Here's how the part is built. I have some questions about the finished solid (model axes, mm). Face numbers are marked on the shaded views. A direction names the side the tool comes from. Give positions to 0.01 mm unless a question says otherwise; leave off trailing zeros. Write each loop counter-clockwise with the first axis right and the second up, starting at its lowest first coordinate (ties: lowest second). Pieces come first, ordered by that corner, then holes. Notation, with made-up numbers: (62, -37.5) - (98, -37.5) arc R6 cw to (98, -32.5) - close; hole circle Ø9 at (33.25, 88.5). An arc over 180 degrees is marked (long way). Write each question's results on one line, items separated by ' | '. Start each with the question number.
Item 1: Which directions (+Z, -Z, +X, -X, +Y, -Y) give clear straight access to the entire face, cutting with the end or side of a thin tool? Please do the marked faces 1 and 2.
Item 2: We'd pull the mould along X, two halves only. Please class the marked faces 3, 4 and 5: +X half, -X half, draft (parallel to the pull), parting line (faces both ways), or undercut.
Item 3: Suppose I cut it at A-A on x = 0. List the corners of the cut face in (y, z) for me.
Item 4: Suppose I cut it at C-C on y = 13.5. List the corners of the cut face in (x, z) for me, then the cut area to 3 significant figures.
Item 5: Suppose I cut it at B-B on z = 0. List the corners of the cut face in (x, y) for me.
Item 6: Will these pins go through, and if not, where does the flat tip stop? P1, Ø4, axis at y = 7.5, z = -1.5, coming from the +X side; P2, Ø8, axis at x = -4, y = 35, coming from the +Z side; P3, Ø6, axis at x = 6.5, z = 5.5, coming from the -Y side; P4, Ø2.5, axis at x = 7, z = 0, coming from the -Y side.
Item 7: Suppose I cut it at D-D on x = 7.5. List the corners of the cut face in (y, z) for me, then the cut area to 3 significant figures.
Item 8: Please list where these lines run through material, in increasing order: line 1 along X through (y, z) = (42.1, 0); line 2 along X through (y, z) = (12, 0); line 3 along Y through (x, z) = (5.75, -8).
```python
from build123d import *

# Parameters (mm, degrees)
SKETCH1_R           = 1.5
BOSS_EXTRUDE1_DEPTH = 40
SKETCH2_R           = 10
SKETCH2_R_2         = 1.6
SKETCH2_R_3         = 1.5
BOSS_EXTRUDE2_DEPTH = 3


with BuildPart() as part:
    # Sketch1 → Boss-Extrude1 (new body)
    with BuildSketch(Plane(origin=(0, 0, 0), x_dir=(1, 0, 0), z_dir=(0, 1, 0))):
        with BuildLine():
            Line((2, 2.236067977), (2, -2.236067977))
            ThreePointArc((2, -2.236067977), (-3, 0), (2, 2.236067977))
        make_face()
        with Locations(Location((0, 0, 0), (0, 0, 270))):
            Circle(SKETCH1_R, mode=Mode.SUBTRACT)
    extrude(amount=BOSS_EXTRUDE1_DEPTH)

    # Sketch2 → Boss-Extrude2 (add)
    with BuildSketch(Plane(origin=(0, 40, 0), x_dir=(1, 0, 0), z_dir=(0, 1, 0))):
        with Locations(Location((0, 0, 0), (0, 0, 270))):
            Circle(SKETCH2_R)
        with Locations(Location((-7, 0, 0), (0, 0, 270))):
            Circle(SKETCH2_R_2, mode=Mode.SUBTRACT)
        with Locations(Location((7, 0, 0), (0, 0, 270))):
            Circle(SKETCH2_R_2, mode=Mode.SUBTRACT)
        with Locations(Location((0, 0, 0), (0, 0, 270))):
            Circle(SKETCH2_R_3, mode=Mode.SUBTRACT)
    extrude(amount=BOSS_EXTRUDE2_DEPTH)


solid = part.part
```
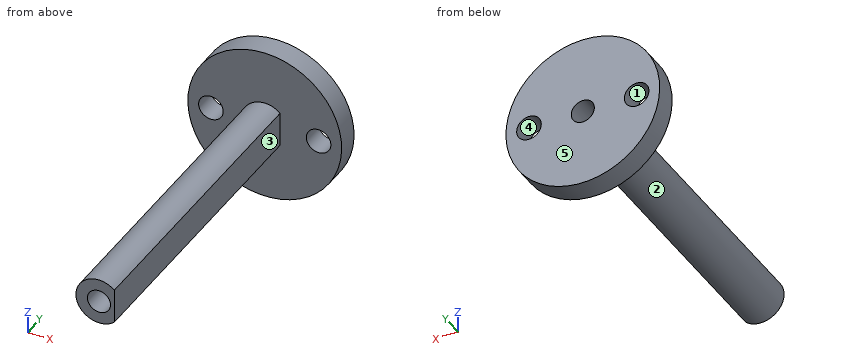
Checked values:
1) face 1: +Y, -Y | face 2: -Y
2) face 3: +X half | face 4: undercut | face 5: draft
3) outline: (0, -3) - (40, -3) - (40, -10) - (43, -10) - (43, -1.5) - (0, -1.5) - close; (0, 1.5) - (43, 1.5) - (43, 10) - (40, 10) - (40, 3) - (0, 3) - close
4) outline: (2, -2.24) - (2, 2.24) arc R3 ccw (long way) to start; hole circle Ø3 at (0, 0) | area: 18.1 mm^2
5) outline: (-10, 40) - (-8.6, 40) - (-8.6, 43) - (-10, 43) - close; (-5.4, 40) - (-3, 40) - (-3, 0) - (-1.5, 0) - (-1.5, 43) - (-5.4, 43) - close; (1.5, 0) - (2, 0) - (2, 40) - (5.4, 40) - (5.4, 43) - (1.5, 43) - close; (8.6, 40) - (10, 40) - (10, 43) - (8.6, 43) - close
6) P1: stops at x = 2 | P2: stops at z = 3 | P3: stops at y = 40 | P4: passes through
7) outline: (40, -6.61) - (43, -6.61) - (43, -1.52) - (40, -1.52) - close; (40, 1.52) - (43, 1.52) - (43, 6.61) - (40, 6.61) - close | area: 30.6 mm^2
8) line 1: x = -10 to -8.6, -5.4 to -1.5, 1.5 to 5.4, 8.6 to 10 | line 2: x = -3 to -1.5, 1.5 to 2 | line 3: y = 40 to 43
